Answer from the drawing. Dimensions are ordinates in mm from the lowest x, y and z of the part. Give positions to 0.01 mm unless a question says otherwise; leave off trailing zeros. Write each loop counter-clockwise with the first axis right and the second up, starting at its lowest first coordinate (ties: lowest second). Pieces come first, ordered by that corner, then holes. Notation, with made-up numbers: (57.5, 45) - (108.5, 45) arc R15 ccw to (108.5, 65) - close; hole circle Ø4 at (48.5, 80). An arc over 180 degrees is marked (long way). Answer as a JSON object with one key per item and string values. Group by question number.
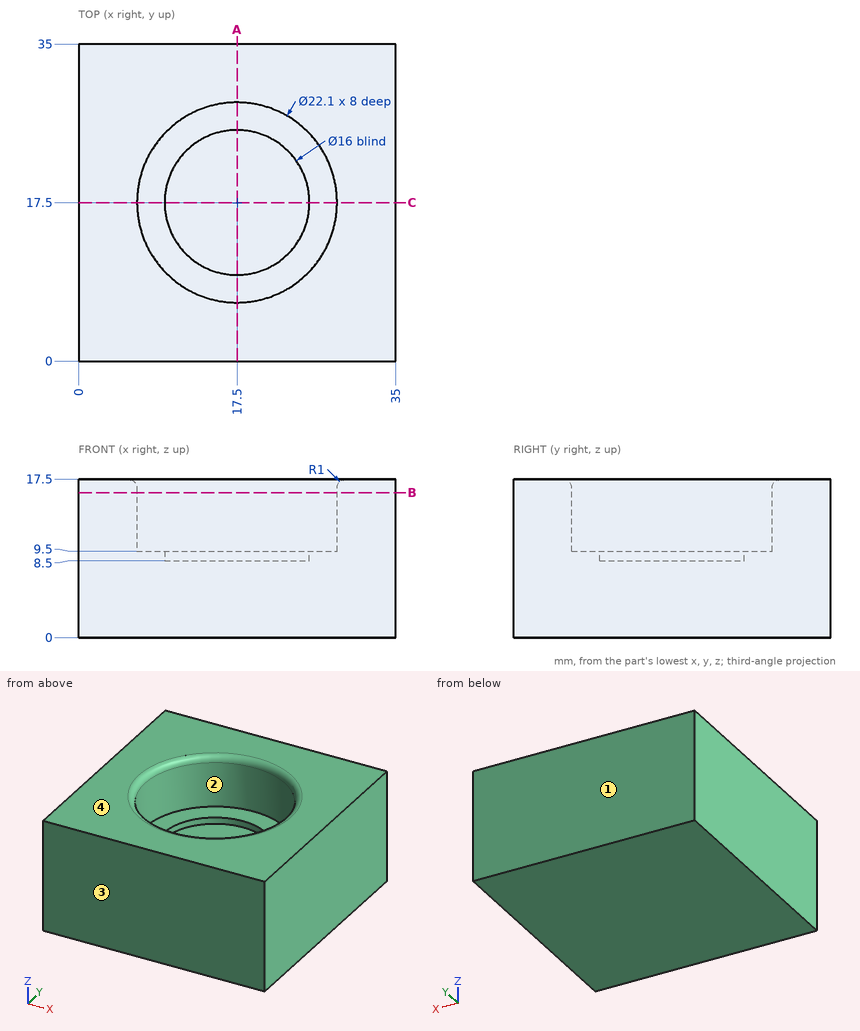
1) For a pull along Y with two mould halves and no side action, classify the marked faces 1, 2, 3 and 4 as released by +Y, released by -Y, zero draft, split by the parting line, or undercut.
2) Find the intervals of material crossed by line 1 (Y direction, x = 17.5, z = 13.75); line 2 (X direction, y = 17.5, z = 8.8), in increasing order. Write a range as [from, to].
3) Flat-ended cylindrical pins translate along their axes: pin 1 Ø5 at (x, y) = (19.5, 15) entering from +Z; pin 2 Ø18.5 at (x, y) = (17.5, 17.5) entering from +Z. Find the tip coordinate at first contact, or state that the pin passes through.
4) Find section A-A, the plane x = 17.5. Write down the section's boundary in (y, z).
5) Find section B-B, the plane z = 16. Write down the section's boundary in (x, y).
Values follow:
{
 "1": {"face 1": "released by +Y", "face 2": "undercut", "face 3": "released by -Y", "face 4": "zero draft"},
 "2": {"line 1": "y = [0, 6.45], [28.55, 35]", "line 2": "x = [0, 9.5], [25.5, 35]"},
 "3": {"pin 1": "stops at z = 8.5", "pin 2": "stops at z = 9.5"},
 "4": {"outline": "(0, 0) - (35, 0) - (35, 17.5) - (29.55, 17.5) arc R1 ccw to (28.55, 16.5) - (28.55, 9.5) - (25.5, 9.5) - (25.5, 8.5) - (9.5, 8.5) - (9.5, 9.5) - (6.45, 9.5) - (6.45, 16.5) arc R1 ccw to (5.45, 17.5) - (0, 17.5) - close"},
 "5": {"outline": "(0, 0) - (35, 0) - (35, 35) - (0, 35) - close; hole circle Ø22.1 at (17.5, 17.5)"}
}
